Check sheet for the modelled part. Datum: model origin and axes. Units: mm. Face numbers are marked on the shaded views. A direction names the side the tool comes from. Give positions to 0.01 mm unless a question says otherwise; leave off trailing zeros. Loops run counter-clockwise (first coordinate to the right, second up) from the corner with the lowest first, then second, coordinate; pieces in that order, holes last. Notation, with made-up numbers: M 83,-15 L 118,-15 A32 ccw 118,12 Z; hole C 29.25,1 d9. An arc over 180 degrees is marked long. Put each result on its own line as item: value. Start each with the question number.
```python
from build123d import *

# Parameters (mm, degrees)
EXTRU_MINCE1_DEPTH      = 33.5
ESQUISSE2_R             = 1.25
ESQUISSE2_W             = 41
ESQUISSE2_H             = 18
ENL_V_MAT_EXTRU_1_DEPTH = 2


with BuildPart() as part:
    # Esquisse1 → Extru.-Mince1 (new, symmetric)
    with BuildSketch(Plane.XY):
        Polygon((0, 20), (0, 0), (30, 0), (30, 2), (2, 2), (2, 20), align=None)
    extrude(amount=EXTRU_MINCE1_DEPTH, both=True)

    # Esquisse2 → Enlèv. mat.-Extru.1 (cut)
    with BuildSketch(Plane.ZY):
        with Locations((-24, 7)):
            Circle(ESQUISSE2_R)
        with Locations((24, 7)):
            Circle(ESQUISSE2_R)
        with Locations((24, 17)):
            Circle(ESQUISSE2_R)
        with Locations((-24, 17)):
            Circle(ESQUISSE2_R)
        with Locations((0, 11)):
            Rectangle(ESQUISSE2_W, ESQUISSE2_H)
    extrude(amount=-ENL_V_MAT_EXTRU_1_DEPTH, mode=Mode.SUBTRACT)


solid = part.part
```
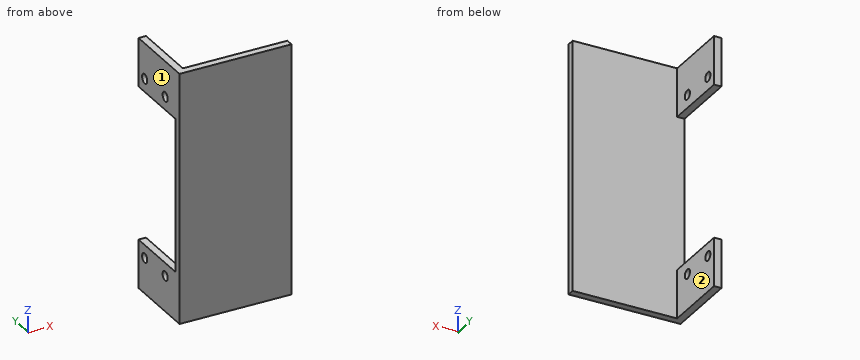
Q1. Section check C-C, the plane x = 14.75. Record the cut outline in (y, z).
Q2. Section check A-A, the plane y = 9.5. Record the cut outline in (x, z), then the cut area to 3 significant figures.
Q3. Access from +Z, -Z, +X, -X, +Y, -Y to the whole of each face (thin tool, end or side, straight path). Record for the marked faces 1 and 2.
Q4. Section check D-D, the plane z = -15.5. Record the cut outline in (x, y), then the cut area to 3 significant figures.
Q5. Depth check by flat-ended pin: P1, Ø4, axis at y = 9, z = 27, coming from the +X side; P2, Ø3, axis at x = 15, z = -4, coming from the +Y side. Enter the tip coordinate at first touch or a pass-through.
Q6. Section check B-B, the plane z = 24. Record the cut outline in (x, y), then the cut area to 3 significant figures.
Q7. Thickness scan on line 1 along Y through (x, z) = (26, -9.5). Record the ranges inside material, lowest first. Write a range as [from, to].
Found:
1. outline: M 0,-33.5 L 2,-33.5 L 2,33.5 L 0,33.5 Z
2. outline: M 0,-33.5 L 2,-33.5 L 2,-20.5 L 0,-20.5 Z; M 0,20.5 L 2,20.5 L 2,33.5 L 0,33.5 Z
2. area: 52.0 mm^2
3. face 1: +Z, -Z, -X, +Y, -Y
3. face 2: +Z, -Z, +X, +Y
4. outline: M 0,0 L 30,0 L 30,2 L 0,2 Z
4. area: 60.0 mm^2
5. P1: stops at x = 2
5. P2: stops at y = 2
6. outline: M 0,0 L 30,0 L 30,2 L 2,2 L 2,5.75 L 0,5.75 Z; M 0,8.25 L 2,8.25 L 2,15.75 L 0,15.75 Z; M 0,18.25 L 2,18.25 L 2,20 L 0,20 Z
6. area: 86.0 mm^2
7. line 1: y = [0, 2]
